Can you work these out from the model? Positions are in its coordinate system, mm. Give positions to 0.01 mm unless a question says otherwise; leave off trailing zeros. Write each loop counter-clockwise with the first axis right and the second up, starting at its lowest first coordinate (ties: lowest second). Pieces come first, ordered by that corner, then holes.
```python
from build123d import *

# Parameters (mm, degrees)
F0_W     = 6.35
F0_H     = 6.35
F3_DEPTH = 11.43
F4_DEPTH = 50.8
F5_DEPTH = 50.8


with BuildPart() as f3:
    # F0 (on Front) → F3 (new body)
    with BuildSketch(Plane.XZ):
        with BuildLine():
            ThreePointArc((50.700684167, 3.175), (50.7751649711, 1.5882764743), (50.8, 0))
            Line((50.8, 0), (50.8, 3.175))
            Line((50.8, 3.175), (50.700684167, 3.175))
        make_face()
        with BuildLine():
            ThreePointArc((-1.86e-08, 50.8), (1.588276465, 50.7751649714), (3.175, 50.700684167))
            Line((3.175, 50.700684167), (3.175, 50.8))
            Line((3.175, 50.8), (-1.86e-08, 50.8))
        make_face()
        with BuildLine():
            ThreePointArc((-3.175, 50.700684167), (-1.5882764835, 50.7751649708), (-1.86e-08, 50.8))
            Line((-1.86e-08, 50.8), (-3.175, 50.8))
            Line((-3.175, 50.8), (-3.175, 50.700684167))
        make_face()
        with BuildLine():
            ThreePointArc((-50.8, -4.94e-08), (-50.7751649719, 1.5882764495), (-50.700684167, 3.175))
            Line((-50.700684167, 3.175), (-50.8, 3.175))
            Line((-50.8, 3.175), (-50.8, -4.94e-08))
        make_face()
        with BuildLine():
            Line((-50.8, -3.175), (-50.700684167, -3.175))
            ThreePointArc((-50.700684167, -3.175), (-50.7751649703, -1.588276499), (-50.8, -4.94e-08))
            Line((-50.8, -4.94e-08), (-50.8, -3.175))
        make_face()
        with BuildLine():
            Line((-3.175, -50.8), (-5.98e-08, -50.8))
            ThreePointArc((-5.98e-08, -50.8), (-1.5882765041, -50.7751649702), (-3.175, -50.700684167))
            Line((-3.175, -50.700684167), (-3.175, -50.8))
        make_face()
        with BuildLine():
            Line((3.175, -50.8), (3.175, -50.700684167))
            ThreePointArc((3.175, -50.700684167), (1.5882764444, -50.775164972), (-5.98e-08, -50.8))
            Line((-5.98e-08, -50.8), (3.175, -50.8))
        make_face()
        with BuildLine():
            Line((50.8, -3.175), (50.8, 0))
            ThreePointArc((50.8, 0), (50.7751649711, -1.5882764743), (50.700684167, -3.175))
            Line((50.700684167, -3.175), (50.8, -3.175))
        make_face()
        with BuildLine():
            ThreePointArc((3.175, 50.700684167), (35.9210244843, 35.9210244843), (50.700684167, 3.175))
            Line((50.700684167, 3.175), (50.8, 3.175))
            Line((50.8, 3.175), (50.8, 50.8))
            Line((50.8, 50.8), (3.175, 50.8))
            Line((3.175, 50.8), (3.175, 50.700684167))
        make_face()
        with BuildLine():
            ThreePointArc((-50.700684167, 3.175), (-35.9210244843, 35.9210244843), (-3.175, 50.700684167))
            Line((-3.175, 50.700684167), (-3.175, 50.8))
            Line((-3.175, 50.8), (-50.8, 50.8))
            Line((-50.8, 50.8), (-50.8, 3.175))
            Line((-50.8, 3.175), (-50.700684167, 3.175))
        make_face()
        with BuildLine():
            Line((-3.175, -50.8), (-3.175, -50.700684167))
            ThreePointArc((-3.175, -50.700684167), (-35.9210244843, -35.9210244843), (-50.700684167, -3.175))
            Line((-50.700684167, -3.175), (-50.8, -3.175))
            Line((-50.8, -3.175), (-50.8, -50.8))
            Line((-50.8, -50.8), (-3.175, -50.8))
        make_face()
        with BuildLine():
            Line((50.8, -3.175), (50.700684167, -3.175))
            ThreePointArc((50.700684167, -3.175), (35.9210244843, -35.9210244843), (3.175, -50.700684167))
            Line((3.175, -50.700684167), (3.175, -50.8))
            Line((3.175, -50.8), (50.8, -50.8))
            Line((50.8, -50.8), (50.8, -3.175))
        make_face()
        with BuildLine():
            ThreePointArc((50.700684167, -3.175), (50.7751649711, -1.5882764743), (50.8, 0))
            ThreePointArc((50.8, 0), (50.7751649711, 1.5882764743), (50.700684167, 3.175))
            Line((50.700684167, 3.175), (3.175, 3.175))
            Line((3.175, 3.175), (3.175, -3.175))
            Line((3.175, -3.175), (50.700684167, -3.175))
        make_face()
        with BuildLine():
            Line((3.175, 3.175), (3.175, 50.700684167))
            ThreePointArc((3.175, 50.700684167), (1.588276465, 50.7751649714), (-1.86e-08, 50.8))
            ThreePointArc((-1.86e-08, 50.8), (-1.5882764835, 50.7751649708), (-3.175, 50.700684167))
            Line((-3.175, 50.700684167), (-3.175, 3.175))
            Line((-3.175, 3.175), (3.175, 3.175))
        make_face()
        with BuildLine():
            Line((-3.175, -3.175), (-3.175, 3.175))
            Line((-3.175, 3.175), (-50.700684167, 3.175))
            ThreePointArc((-50.700684167, 3.175), (-50.7751649719, 1.5882764495), (-50.8, -4.94e-08))
            ThreePointArc((-50.8, -4.94e-08), (-50.7751649703, -1.588276499), (-50.700684167, -3.175))
            Line((-50.700684167, -3.175), (-3.175, -3.175))
        make_face()
        with BuildLine():
            ThreePointArc((-5.98e-08, -50.8), (1.5882764444, -50.775164972), (3.175, -50.700684167))
            Line((3.175, -50.700684167), (3.175, -3.175))
            Line((3.175, -3.175), (-3.175, -3.175))
            Line((-3.175, -3.175), (-3.175, -50.700684167))
            ThreePointArc((-3.175, -50.700684167), (-1.5882765041, -50.7751649702), (-5.98e-08, -50.8))
        make_face()
        with BuildLine():
            Line((3.175, 3.175), (50.700684167, 3.175))
            ThreePointArc((50.700684167, 3.175), (35.9210244843, 35.9210244843), (3.175, 50.700684167))
            Line((3.175, 50.700684167), (3.175, 3.175))
        make_face()
        with BuildLine():
            Line((-50.700684167, 3.175), (-3.175, 3.175))
            Line((-3.175, 3.175), (-3.175, 50.700684167))
            ThreePointArc((-3.175, 50.700684167), (-35.9210244843, 35.9210244843), (-50.700684167, 3.175))
        make_face()
        with BuildLine():
            ThreePointArc((3.175, -50.700684167), (35.9210244843, -35.9210244843), (50.700684167, -3.175))
            Line((50.700684167, -3.175), (3.175, -3.175))
            Line((3.175, -3.175), (3.175, -50.700684167))
        make_face()
        with BuildLine():
            Line((-3.175, -50.700684167), (-3.175, -3.175))
            Line((-3.175, -3.175), (-50.700684167, -3.175))
            ThreePointArc((-50.700684167, -3.175), (-35.9210244843, -35.9210244843), (-3.175, -50.700684167))
        make_face()
        Rectangle(F0_W, F0_H)
    extrude(amount=-F3_DEPTH)

    # F1 (on Right) → F4 (cut, symmetric)
    with BuildSketch(Plane.YZ):
        Polygon((6.35, 6.604), (0, 3.175), (0, -3.175), (6.35, -6.604), (6.35, 0), align=None)
    extrude(amount=F4_DEPTH, both=True, mode=Mode.SUBTRACT)

    # F2 (on Top) → F5 (cut, symmetric)
    with BuildSketch(Plane.XY):
        Polygon((-6.604, 6.35), (-3.175, 0), (3.175, 0), (6.604, 6.35), (0, 6.35), align=None)
    extrude(amount=F5_DEPTH, both=True, mode=Mode.SUBTRACT)


solid = f3.part
```
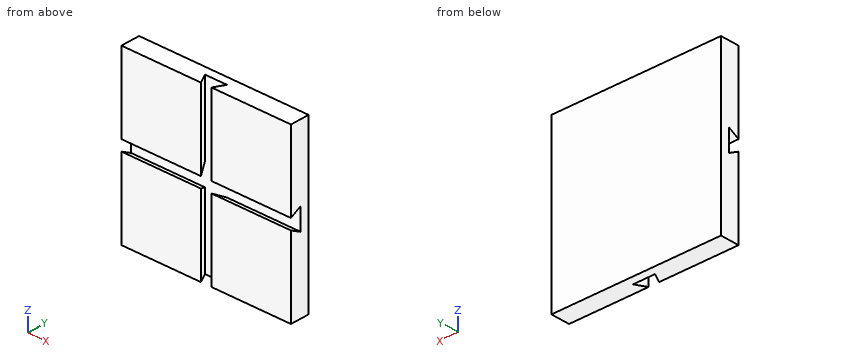
1) Suppose I cut it at B-B on z = -21. Write out the boundary of the cut face in (x, y) (3 decimals), plus the area to 3 significant figures.
Values follow:
outline: (-50.8, 0) - (-3.175, 0) - (-6.604, 6.35) - (6.604, 6.35) - (3.175, 0) - (50.8, 0) - (50.8, 11.43) - (-50.8, 11.43) - close
area: 1,100 mm2
2) Please list where these lines run through material, in increasing order: L1, parallel to X at y = 1.75, z = 16.5; L2, parallel to X at y = 4.75, z = -22; L3, parallel to Y at x = -4, z = 46.
Values follow:
L1: x = -50.8 to -4.12, 4.12 to 50.8
L2: x = -50.8 to -5.74, 5.74 to 50.8
L3: y = 0 to 1.53, 6.35 to 11.43
3) Suppose I cut it at A-A on y = 2.75. Write out the boundary of the cut face in (x, z), plus the area to 3 significant figures.
Values follow:
outline: (-50.8, -50.8) - (-4.66, -50.8) - (-4.66, -4.66) - (-50.8, -4.66) - close; (-50.8, 4.66) - (-4.66, 4.66) - (-4.66, 50.8) - (-50.8, 50.8) - close; (4.66, -50.8) - (50.8, -50.8) - (50.8, -4.66) - (4.66, -4.66) - close; (4.66, 4.66) - (50.8, 4.66) - (50.8, 50.8) - (4.66, 50.8) - close
area: 8,520 mm2
4) Suppose I cut it at C-C on x = -36. Write out the boundary of the cut face in (y, z) (3 decimals), plus the area to 3 significant figures.
Values follow:
outline: (0, -50.8) - (11.43, -50.8) - (11.43, 50.8) - (0, 50.8) - (0, 3.175) - (6.35, 6.604) - (6.35, -6.604) - (0, -3.175) - close
area: 1,100 mm2
